Model file for the job. Use its own axes, mm. Face numbers are marked on the shaded views. A direction names the side the tool comes from. Coordinates: 2 decimals unless noted, no trailing zeros. Write each loop counter-clockwise with the first axis right and the second up, starting at its lowest first coordinate (ties: lowest second). Pieces come first, ordered by that corner, then holes. Notation, with made-up numbers: M -28.75,-17 L 3.25,-17 A11 ccw 3.25,-12 Z; hole C 56.25,45.5 d9. An arc over 180 degrees is marked long. Use CSV: the item, a comma, the result in double quotes. Start each with the question number.
Autodesk Inventor part; units mm, degrees
ref_plane "YZ Plane" through (0, 0, 0) normal (1, 0, 0) x (0, 1, 0)
ref_plane "XZ Plane" through (0, 0, 0) normal (0, 1, 0) x (-1, 0, 0)
ref_plane "XY Plane" through (0, 0, 0) normal (0, 0, 1) x (1, 0, 0)
sketch "Szkic1" plane through (0, 0, 0) normal (0, 1, 0) x (-1, 0, 0)
  circle A0 centre (0, 0) radius 5
  line L0 (1.4434, 2.5) -> (2.8868, 0)
  line L1 (2.8868, 0) -> (1.4434, -2.5)
  line L2 (1.4434, -2.5) -> (-1.4434, -2.5)
  line L3 (-1.4434, -2.5) -> (-2.8868, 0)
  line L4 (-2.8868, 0) -> (-1.4434, 2.5)
  line L5 (-1.4434, 2.5) -> (1.4434, 2.5)
  circle A1 centre (0, 0) radius 3
  dimension "d0" = 10
  dimension "d1" = 5
  dimension "d2" = 6
extrude "Wyciągnięcie proste1" add sketch "Szkic1" along normal blind 2 contours A0 | L0 L1 L2 L3 L4 L5 | A1
extrude "Wyciągnięcie proste2" add sketch "Szkic1" against normal blind 4 contours A0 | A1
sketch "Szkic2" plane through (0, 2, 0) normal (0, 1, 0) x (1, 0, 0)
  circle A0 centre (0, 0) radius 3
  dimension "d7" = 6
extrude "Wyciągnięcie proste3" add sketch "Szkic2" along normal blind 35
thread "Gwint1"
properties part number "M6x35"
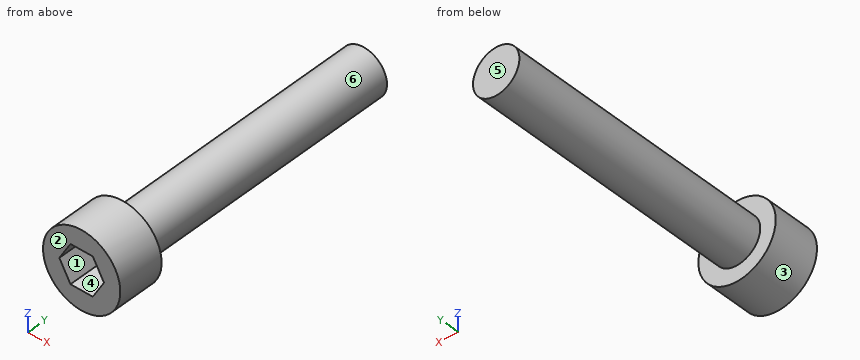
1) Band-saw the part on C-C on y = 27.5. List the corners of the cut face in (x, z).
2) Band-saw the part on A-A on x = 0. List the corners of the cut face in (y, z).
3) Tool access for the marked faces 5 and 6: list every direction of +Z, -Z, +X, -X, +Y, -Y with a clear straight run to the whole face (end or side of a thin tool).
4) Drop flat-ended pins along their axis: P1, Ø4, axis at y = 16.5, z = 0, coming from the +X side; P2, Ø1, axis at x = -3, y = 33, coming from the -Z side; P3, Ø3, axis at x = -2, y = 17, coming from the -Z side. Give the stop position or say it passes through.
5) Two-plate mould, pull along X, no slides. Class the marked faces 1, 2, 3 and 4: pulls with the +X half, pulls with the -X half, needs draft (parallel to the pull), parting line crosses it, or undercut.
6) Band-saw the part on B-B on z = -1.5. List the corners of the cut face in (x, y), then the cut area to 3 significant figures.
7) Wall check: L1, parallel to Y at x = 1.5, z = -3.5; L2, parallel to Z at x = 0, y = 28; L3, parallel to Y at x = 1.75, z = -1. Give the ranges that are in metal, low to high. Write a range as [from, to].
Findings below:
1,outline,"C 0,0 d6"
2,outline,"M -4,-5 L 2,-5 L 2,-3 L 37,-3 L 37,3 L 2,3 L 2,5 L -4,5 L -4,2.5 L 0,2.5 L 0,-2.5 L -4,-2.5 Z"
3,face 5,"+Z, -Z, +X, -X, +Y"
3,face 6,"+Y"
4,P1,"stops at x = 3"
4,P2,"stops at z = -1.66"
4,P3,"stops at z = -2.96"
5,face 1,"undercut"
5,face 2,"needs draft"
5,face 3,"parting line crosses it"
5,face 4,"undercut"
6,outline,"M -4.77,-4 L -2.02,-4 L -2.02,0 L 2.02,0 L 2.02,-4 L 4.77,-4 L 4.77,2 L 2.6,2 L 2.6,37 L -2.6,37 L -2.6,2 L -4.77,2 Z"
6,area,"223 mm2"
7,L1,"y = [-4, 2]"
7,L2,"z = [-3, 3]"
7,L3,"y = [0, 37]"
